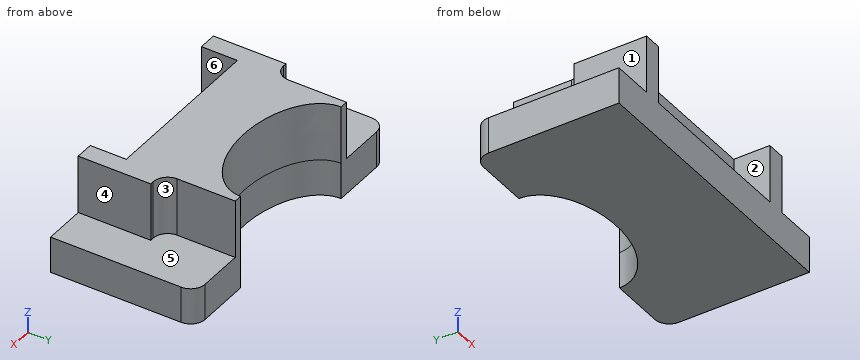
from build123d import *

# Parameters (mm, degrees)
F1_DEPTH = 6.35
F3_DEPTH = 10.16
F4_R     = 2.54


with BuildPart() as f1:
    # F0 (on Top) → F1 (new body)
    with BuildSketch(Plane.XY):
        with BuildLine():
            Line((25.4, -12.7), (25.4, 12.7))
            Line((25.4, 12.7), (13.4078692645, 12.7))
            add(Edge.make_bspline(
                [(-13.4078692645, 12.7), (-13.4078692645, 4.5109884671), (0, 4.5109884671), (13.4078692645, 4.5109884671), (13.4078692645, 12.7)],
                knots=[3.1415926536, 3.1415926536, 3.1415926536, 4.7123889804, 4.7123889804, 6.2831853072, 6.2831853072, 6.2831853072], degree=2, weights=[1, 0.7071067812, 1, 0.7071067812, 1]))
            Line((-13.4078692645, 12.7), (-25.4, 12.7))
            Line((-25.4, 12.7), (-25.4, -12.7))
            Line((-25.4, -12.7), (25.4, -12.7))
        make_face()
    extrude(amount=F1_DEPTH)

    # F2 (on face) → F3 (join)
    with BuildSketch(Plane.XY.offset(6.35)):
        with BuildLine():
            Line((-18.0192738771, -6.3928803429), (-18.0192738771, -12.7))
            Line((-18.0192738771, -12.7), (-14.8282703012, -12.7))
            Line((-14.8282703012, -12.7), (-14.8282703012, -6.3928803429))
            Line((-14.8282703012, -6.3928803429), (0, -6.3928803429))
            Line((0, -6.3928803429), (14.8282703012, -6.3928803429))
            Line((14.8282703012, -6.3928803429), (14.8282703012, -12.7))
            Line((14.8282703012, -12.7), (18.0192738771, -12.7))
            Line((18.0192738771, -12.7), (18.0192738771, -6.3928803429))
            Line((18.0192738771, -6.3928803429), (18.0192738771, 0))
            Line((18.0192738771, 0), (14.8282703012, 0))
            Line((14.8282703012, 0), (14.8282703012, 12.7))
            Line((14.8282703012, 12.7), (13.4078692645, 12.7))
            add(Edge.make_bspline(
                [(-13.4078692645, 12.7), (-13.4078692645, 4.5109884671), (0, 4.5109884671), (13.4078692645, 4.5109884671), (13.4078692645, 12.7)],
                knots=[3.1415926536, 3.1415926536, 3.1415926536, 4.7123889804, 4.7123889804, 6.2831853072, 6.2831853072, 6.2831853072], degree=2, weights=[1, 0.7071067812, 1, 0.7071067812, 1]))
            Line((-13.4078692645, 12.7), (-14.8282703012, 12.7))
            Line((-14.8282703012, 12.7), (-14.8282703012, 0))
            Line((-14.8282703012, 0), (-18.0192738771, 0))
            Line((-18.0192738771, 0), (-18.0192738771, -6.3928803429))
        make_face()
    extrude(amount=F3_DEPTH)

    # F4
    f4_edges = [f1.edges().sort_by_distance(p)[0] for p in [
        (14.82827, 0, 11.43),
        (-14.82827, 0, 11.43),
        (25.4, 12.7, 3.175),
        (-25.4, 12.7, 3.175),
    ]]
    fillet(f4_edges, radius=F4_R)


solid = f1.part
Geometry check sheet. Reference: the model listing, model coordinates, mm. Face numbers are marked on the shaded views. A direction names the side the tool comes from. Coordinates: 2 decimals unless noted, no trailing zeros. Loops run counter-clockwise (first coordinate to the right, second up) from the corner with the lowest first, then second, coordinate; pieces in that order, holes last. Notation, with made-up numbers: (-24.5, 48) - (4.5, 48) arc R23 cw to (4.5, 58) - close; hole circle Ø4 at (-20.75, 15). An arc over 180 degrees is marked (long way). Use one line per item in the form item = value. Start each with the question number.
Item 1: Section check B-B, the plane x = 20. Enter the section's corners in (y, z).
Item 2: Mould release check, pull along X, two halves, no side actions. Record for the marked faces 4, 5 and 6: +X half, -X half, draft (parallel to the pull), parting line (faces both ways), or undercut.
Item 3: Section check C-C, the plane y = -2.25. Enter the section's corners in (x, z), and give its area (3 significant figures).
Item 4: Section check A-A, the plane y = -7.75. Enter the section's corners in (x, z), and give its area (3 significant figures).
Item 5: Tool access check on the marked faces 1, 2 and 3. Record the directions out of +Z, -Z, +X, -X, +Y, -Y that give a thin tool (end or side, any length) a straight path to the whole face; none if there is none.
Item 6: Thickness scan on probe 1 along X at (y, z) = (-7.5, 14); probe 2 along Z at (x, y) = (21, -9); probe 3 along X at (y, z) = (-2.5, 8.5). Record the ranges inside material, lowest first.
Item 7: Section check D-D, the plane x = -16.5. Enter the section's corners in (y, z), and give its area (3 significant figures).
Item 8: Gauge pin test, flat ends, axial feed: pin 1 (1 mm diameter, centred on y = -7.5, z = 7.5, fed in from +X); pin 2 (12 mm diameter, centred on x = 12.5, y = 6.5, fed in from -Z); pin 3 (3 mm diameter, centred on y = -9.5, z = 13.5, fed in from -X); pin 4 (5 mm diameter, centred on x = -5.5, y = -9, fed in from +Z). Record the tip position at first contact, or that the pin passes through.
Computed:
q1.outline = (-12.7, 0) - (12.7, 0) - (12.7, 6.35) - (-12.7, 6.35) - close
q2.face_4 = +X half
q2.face_5 = draft
q2.face_6 = undercut
q3.outline = (-25.4, 0) - (25.4, 0) - (25.4, 6.35) - (18.02, 6.35) - (18.02, 16.51) - (-18.02, 16.51) - (-18.02, 6.35) - (-25.4, 6.35) - close
q3.area = 689 mm2
q4.outline = (-25.4, 0) - (25.4, 0) - (25.4, 6.35) - (18.02, 6.35) - (18.02, 16.51) - (14.83, 16.51) - (14.83, 6.35) - (-14.83, 6.35) - (-14.83, 16.51) - (-18.02, 16.51) - (-18.02, 6.35) - (-25.4, 6.35) - close
q4.area = 387 mm2
q5.face_1 = +Z, -X, +Y, -Y
q5.face_2 = +Z, -Y
q5.face_3 = +Z, +X, +Y
q6.probe_1 = -18.02 to -14.83, 14.83 to 18.02
q6.probe_2 = 0 to 6.35
q6.probe_3 = -18.02 to 18.02
q7.outline = (-12.7, 0) - (12.7, 0) - (12.7, 6.35) - (0.15, 6.35) - (0.15, 16.51) - (-12.7, 16.51) - close
q7.area = 292 mm2
q8.pin_1 = 18.02
q8.pin_2 = 0
q8.pin_3 = -18.02
q8.pin_4 = 6.35
